The listing builds one solid part. Answer for the finished solid, in the listing's coordinates (mm). A direction names the side the tool comes from. Give positions to 0.01 mm unless a question says otherwise; leave off trailing zeros. Order: outer loops, then holes, each group sorted by start corner. A loop starts at its lowest first (then second) coordinate and runs counter-clockwise, first axis right, second up. Notation, with made-up numbers: (89.25, -35) - (105.25, -35) arc R15 cw to (105.25, -28) - close; hole circle Ø10 at (83.5, -19). An arc over 180 degrees is marked (long way). Answer in a Markdown table with one row per item.
from build123d import *

# Parameters (mm, degrees)
F0_W           = 69.5
F0_H           = 55
F1_DEPTH       = 33
F2_SIZE        = 0.5
F4_D           = 17.5
F4_DEPTH       = 23
F4_TIP         = 5.2575304165
F5_D           = 15
F5_DEPTH       = 26.5
F5_TIP         = 4.5064546427
F8_D           = 4
F8_DEPTH       = 54.5
F8_CBORE_D     = 10
F8_CBORE_DEPTH = 1.5
F8_TIP         = 1.2017212381
F9_D           = 4.2
F9_DEPTH       = 15
F9_TIP         = 1.2618073
F10_D          = 3
F10_DEPTH      = 8
F10_TIP        = 0.9012909285
F11_D          = 3
F11_DEPTH      = 8
F11_TIP        = 0.9012909285
F12_D          = 4.2
F12_DEPTH      = 17
F12_TIP        = 1.2618073


with BuildPart() as f1:
    # F0 (on Front) → F1 (new body)
    with BuildSketch(Plane.XZ):
        with Locations((34.75, 27.5)):
            Rectangle(F0_W, F0_H)
    extrude(amount=-F1_DEPTH)

    # F2
    f2_edges = [f1.edges().sort_by_distance(p)[0] for p in [
        (0, 0, 27.5),
        (34.75, 0, 0),
        (69.5, 0, 27.5),
        (34.75, 0, 55),
        (0, 33, 27.5),
        (34.75, 33, 0),
        (69.5, 33, 27.5),
        (34.75, 33, 55),
        (69.5, 16.5, 55),
        (0, 16.5, 55),
        (0, 16.5, 0),
        (69.5, 16.5, 0),
    ]]
    chamfer(f2_edges, length=F2_SIZE)

    # F4
    with Locations(Plane.XZ):
        with Locations((15, 39)):
            Hole(F4_D / 2, depth=F4_DEPTH)
            with Locations((0, 0, -(F4_DEPTH + F4_TIP / 2))):  # 118° drill point
                Cone(0, F4_D / 2, F4_TIP, mode=Mode.SUBTRACT)

    # F5
    with Locations(Plane.XZ):
        with Locations((15, 39)):
            Hole(F5_D / 2, depth=F5_DEPTH)
            with Locations((0, 0, -(F5_DEPTH + F5_TIP / 2))):  # 118° drill point
                Cone(0, F5_D / 2, F5_TIP, mode=Mode.SUBTRACT)

    # F8
    with Locations(Plane.YZ.offset(69.5)):
        with Locations((26.5, 39)):
            CounterBoreHole(F8_D / 2, F8_CBORE_D / 2, F8_CBORE_DEPTH, depth=F8_DEPTH)
            with Locations((0, 0, -(F8_DEPTH + F8_TIP / 2))):  # 118° drill point
                Cone(0, F8_D / 2, F8_TIP, mode=Mode.SUBTRACT)

    # F9
    with Locations(Plane.YZ.offset(69.5)):
        with Locations((14, 49), (14, 29)):
            Hole(F9_D / 2, depth=F9_DEPTH)
            with Locations((0, 0, -(F9_DEPTH + F9_TIP / 2))):  # 118° drill point
                Cone(0, F9_D / 2, F9_TIP, mode=Mode.SUBTRACT)

    # F10
    with Locations(Plane.YZ.offset(69.5)):
        with Locations((6, 49), (6, 29)):
            Hole(F10_D / 2, depth=F10_DEPTH)
            with Locations((0, 0, -(F10_DEPTH + F10_TIP / 2))):  # 118° drill point
                Cone(0, F10_D / 2, F10_TIP, mode=Mode.SUBTRACT)

    # F11
    with Locations(Plane(origin=(0, 0, 0), x_dir=(1, 0, 0), z_dir=(0, 0, -1))):
        with Locations((9, -24), (60, -6)):
            Hole(F11_D / 2, depth=F11_DEPTH)
            with Locations((0, 0, -(F11_DEPTH + F11_TIP / 2))):  # 118° drill point
                Cone(0, F11_D / 2, F11_TIP, mode=Mode.SUBTRACT)

    # F12
    with Locations(Plane(origin=(0, 0, 0), x_dir=(1, 0, 0), z_dir=(0, 0, -1))):
        with Locations((29, -16.5), (59, -16.5)):
            Hole(F12_D / 2, depth=F12_DEPTH)
            with Locations((0, 0, -(F12_DEPTH + F12_TIP / 2))):  # 118° drill point
                Cone(0, F12_D / 2, F12_TIP, mode=Mode.SUBTRACT)


solid = f1.part
Item 1: Determine the mould class of faces 4 (the face through (60.241, 6.1, 8.745)), 5 (the face through (10.96, 11.66, 31.24)), 6 (the face through (69.5, 16, 27)), 7 (the face through (34, 16, 55)) for opening direction Z: pulls with the +Z half, pulls with the -Z half, needs draft (parallel to the pull), parting line crosses it, or undercut.
Answer block:
| item | result |
|---|---|
| face 4 | pulls with the -Z half |
| face 5 | undercut |
| face 6 | needs draft |
| face 7 | pulls with the +Z half |
Item 2: Which of the six approach directions +Z, -Z, +X, -X, +Y, -Y give full straight-line access (tool end or side, diameter ignored) to faces 1 (the face through (68.76, 22.815, 42.379)), 2 (the face through (0, 16, 27)), 3 (the face through (30.548, 15.081, 8.619))?
Answer block:
| item | result |
|---|---|
| face 1 | +X |
| face 2 | +Z, -Z, -X, +Y, -Y |
| face 3 | -Z |
Item 3: Find section A-A on z = 6. Write down the section's boundary in (x, y).
Answer block:
| item | result |
|---|---|
| outline | (0, 0.5) - (0.5, 0) - (69, 0) - (69.5, 0.5) - (69.5, 32.5) - (69, 33) - (0.5, 33) - (0, 32.5) - close; hole circle Ø3 at (9, 24); hole circle Ø4.2 at (29, 16.5); hole circle Ø4.2 at (59, 16.5); hole circle Ø3 at (60, 6) |
Item 4: Consider line 1 (Y direction, x = 67.5, z = 29); line 2 (X direction, y = 16.5, z = 5.75); line 3 (Y direction, x = 52, z = 39). Determine where each line is inside the solid, lowest interval first.
Answer block:
| item | result |
|---|---|
| line 1 | 0 to 4.5, 7.5 to 11.9, 16.1 to 33 |
| line 2 | 0 to 26.9, 31.1 to 56.9, 61.1 to 69.5 |
| line 3 | 0 to 24.5, 28.5 to 33 |
Item 5: Each of these flat-tipped pins is pushed along its axis until it touches: P1, Ø13, axis at y = 26.5, z = 39, coming from the +X side; P2, Ø4, axis at y = 14, z = 49, coming from the +X side; P3, Ø2.5, axis at y = 14, z = 29, coming from the +X side; P4, Ø1.8, axis at x = 9, y = 24, coming from the -Z side. Where does it stop, or does it pass through?
Answer block:
| item | result |
|---|---|
| P1 | x = 69.5 |
| P2 | x = 54.44 |
| P3 | x = 53.99 |
| P4 | z = 8.36 |
